Check sheet for the modelled part. Datum: model origin and axes. Units: mm. A direction names the side the tool comes from. Give positions to 0.01 mm unless a question says otherwise; leave off trailing zeros. Order: outer loops, then holes, each group sorted by start corner. A loop starts at its lowest first (then second) coordinate and runs counter-clockwise, first axis right, second up.
from build123d import *

# Parameters (mm, degrees)
F0_R     = 32.5
F1_DEPTH = 5
F2_R     = 32.5
F2_R_2   = 30
F3_DEPTH = 25
F4_R     = 2
F5_DEPTH = 25
F6_R     = 1.5
F7_DEPTH = 25
F8_R     = 5
F9_R     = 1


with BuildPart() as f1:
    # F0 (on Top) → F1 (new body)
    with BuildSketch(Plane.XY):
        Circle(F0_R)
    extrude(amount=F1_DEPTH)

    # F2 (on face) → F3 (join)
    with BuildSketch(Plane.XY.offset(5)):
        Circle(F2_R)
        Circle(F2_R_2, mode=Mode.SUBTRACT)
    extrude(amount=F3_DEPTH)

    # F4 (on face) → F5 (cut)
    with BuildSketch(Plane(origin=(0, 0, 0), x_dir=(1, 0, 0), z_dir=(0, 0, -1))):
        Circle(F4_R)
    extrude(amount=-F5_DEPTH, mode=Mode.SUBTRACT)

    # F6 (on face) → F7 (cut)
    with BuildSketch(Plane(origin=(0, 0, 0), x_dir=(1, 0, 0), z_dir=(0, 0, -1))):
        with Locations((0, 25)):
            Circle(F6_R)
        with Locations((17.67767, 17.67767)):
            Circle(F6_R)
        with BuildLine():
            ThreePointArc((23.5, 0), (25, -1.5), (26.5, 0))
            ThreePointArc((26.5, 0), (25, 1.5), (23.5, 0))
        make_face()
        with Locations((17.67767, -17.67767)):
            Circle(F6_R)
        with Locations((0, -25)):
            Circle(F6_R)
        with Locations((-17.67767, -17.67767)):
            Circle(F6_R)
        with Locations((-17.67767, 17.67767)):
            Circle(F6_R)
        with Locations((-25, 0)):
            Circle(F6_R)
    extrude(amount=-F7_DEPTH, mode=Mode.SUBTRACT)

    # F8
    f8_edges = [f1.edges().sort_by_distance(p)[0] for p in [
        (-32.5, 0, 0),
    ]]
    fillet(f8_edges, radius=F8_R)

    # F9
    f9_edges = [f1.edges().sort_by_distance(p)[0] for p in [
        (-30, 0, 30),
        (-32.5, 0, 30),
    ]]
    fillet(f9_edges, radius=F9_R)


solid = f1.part
1) Set-up check for faces 1 (the face through (-29.97, 1.32, 16.83)), 2 (the face through (17.35, 19.14, 2.46)): record each of +Z, -Z, +X, -X, +Y, -Y from which the full face is reachable in a straight line by a thin tool's end or side.
Recorded:
face 1: +Z
face 2: +Z, -Z
2) Material ranges on L1, parallel to Y at x = 0, z = 1.45; L2, parallel to Y at x = 0, z = 3.3; L3, parallel to Y at x = -1, z = 12.75, recorded low to high.
Recorded:
L1: y = -31.02 to -26.5, -23.5 to -2, 2 to 23.5, 26.5 to 31.02
L2: y = -32.2 to -26.5, -23.5 to -2, 2 to 23.5, 26.5 to 32.2
L3: y = -32.48 to -29.98, 29.98 to 32.48
3) Depth check by flat-ended pin: pin 1 Ø1.8 at (x, y) = (0, -25) entering from +Z; pin 2 Ø5 at (y, z) = (-23.5, 4.5) entering from -X; pin 3 Ø1 at (x, z) = (19.5, 7.5) entering from -Y; pin 4 Ø1.5 at (x, y) = (22.5, -18.5) entering from +Z. Enter the tip coordinate at first touch or a pass-through.
Recorded:
pin 1: passes through
pin 2: stops at x = -24.79
pin 3: stops at y = -26.37
pin 4: stops at z = 5
4) Section check C-C, the plane x = 17.5. State how many separate pieces and enclosed holes the cut face has, then the cut area to 3 significant figures.
Recorded:
separate pieces: 3
enclosed holes: 0
area: 381 mm2
5) Draft check along X on faces 3 (the face through (0, 2, 2)), 4 (the face through (31, 9.76, 16.83)), 5 (the face through (0, -6, 0)). Enter one of: +X half, -X half, draft (parallel to the pull), parting line (faces both ways), or undercut.
Recorded:
face 3: undercut
face 4: parting line
face 5: draft
6) Section check A-A, the plane y = 0. Record the cut outline in (x, z).
Recorded:
outline: (-32.5, 5) arc R5 ccw to (-27.5, 0) - (-26.5, 0) - (-26.5, 5) - (-30, 5) - (-30, 29) arc R1 ccw to (-31, 30) - (-31.5, 30) arc R1 ccw to (-32.5, 29) - close; (-23.5, 0) - (-2, 0) - (-2, 5) - (-23.5, 5) - close; (2, 0) - (23.5, 0) - (23.5, 5) - (2, 5) - close; (26.5, 0) - (27.5, 0) arc R5 ccw to (32.5, 5) - (32.5, 29) arc R1 ccw to (31.5, 30) - (31, 30) arc R1 ccw to (30, 29) - (30, 5) - (26.5, 5) - close
7) Section check B-B, the plane z = 24.25. Record the cut outline in (x, y), then the cut area to 3 significant figures.
Recorded:
outline: circle Ø65 at (0, 0); hole circle Ø60 at (0, 0)
area: 491 mm2
